Autodesk Inventor part; units mm, degrees
ref_plane "YZ Plane" through (0, 0, 0) normal (1, 0, 0) x (0, 1, 0)
ref_plane "XZ Plane" through (0, 0, 0) normal (0, 1, 0) x (-1, 0, 0)
ref_plane "XY Plane" through (0, 0, 0) normal (0, 0, 1) x (1, 0, 0)
sketch "Esquisse1" plane through (0, 0, 0) normal (0, 1, 0) x (-1, 0, 0)
  line L0 (28.5, 18.5) -> (-28.5, 18.5)
  line L1 (-28.5, 18.5) -> (-28.5, -18.5)
  line L2 (-28.5, -18.5) -> (28.5, -18.5)
  line L3 (28.5, -18.5) -> (28.5, 18.5)
  line L4 (28.5, 18.5) -> (-28.5, -18.5) construction
  line L5 (-28.5, 18.5) -> (28.5, -18.5) construction
  point P0 (0, 0)
  dimension "d0" = 57
  dimension "d1" = 37
extrude "Extrusion1" add sketch "Esquisse1" along normal blind 23
sketch "Esquisse2" plane through (0, 23, 0) normal (0, 1, 0) x (1, 0, 0)
  line L0 (-28.5, -18.5) -> (28.5, -18.5)
  line L1 (28.5, -18.5) -> (28.5, 18.5)
  line L2 (-28.5, 18.5) -> (-8.5, 18.5)
  line L3 (-8.5, 18.5) -> (-8.5, -18.5)
  line L4 (-8.5, -18.5) -> (-28.5, -18.5)
  line L5 (-28.5, -18.5) -> (-28.5, 18.5)
  line L6 (28.5, 18.5) -> (28.5, 16.5) construction
  line L7 (28.5, -18.5) -> (28.5, -16.5) construction
  line L8 (28.5, 16.5) -> (-8.5, 16.5)
  line L9 (-8.5, 16.5) -> (-8.5, -16.5)
  line L10 (-8.5, -16.5) -> (28.5, -16.5)
  line L11 (28.5, -16.5) -> (28.5, 16.5)
  point P0 (0, 0)
  dimension "d4" = 20
  dimension "d5" = 2
  dimension "d6" = 2
  dimension "d7" = 33
extrude "Extrusion2" cut sketch "Esquisse2" against normal blind 21 contours L3 L8 L1 L10
sketch "Esquisse3" plane through (-8.5, 23, 16.5) normal (1, 0, 0) x (0, 0, -1)
  line L0 (0, 0) -> (0, -21)
  line L1 (33, -21) -> (0, -21)
  line L2 (0, -21) -> (0, -2)
  line L3 (0, -2) -> (33, -2)
  line L4 (33, -2) -> (33, -21)
  point P0 (16.5, -23)
  dimension "d10" = 19
extrude "Extrusion3" cut sketch "Esquisse3" against normal blind 18
sketch "Esquisse4" plane through (-28.5, 0, -18.5) normal (-1, 0, 0) x (0, 0, 1)
  line L0 (37, 0) -> (18.5, 0) construction
  line L1 (18.5, 0) -> (18.5, 11.5) construction
  line L2 (18.5, 11.5) -> (37, 11.5) construction
  line L3 (37, 11.5) -> (37, 0) construction
  line L4 (6.5, 4.25) -> (30.5, 4.25)
  line L5 (30.5, 4.25) -> (30.5, 18.75)
  line L6 (30.5, 18.75) -> (6.5, 18.75)
  line L7 (6.5, 18.75) -> (6.5, 4.25)
  line L8 (6.5, 4.25) -> (30.5, 18.75) construction
  line L9 (30.5, 4.25) -> (6.5, 18.75) construction
  dimension "d13" = 18.5
  dimension "d14" = 11.5
  dimension "d15" = 24
  dimension "d16" = 14.5
extrude "Extrusion4" cut sketch "Esquisse4" against normal blind 5
properties part number "mount pour oeil"
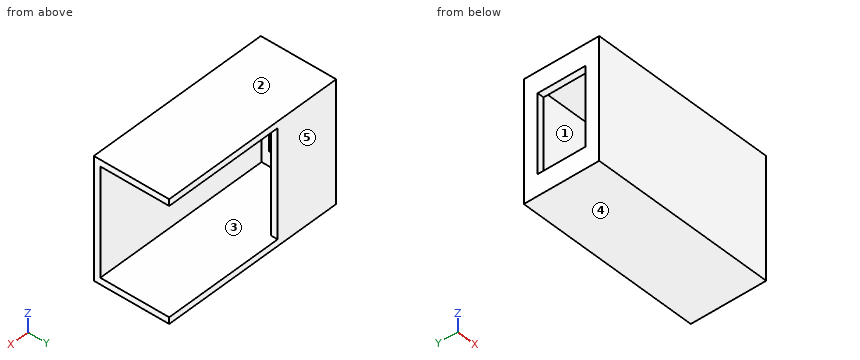
For this review, take the finished solid that the model builds, in its own axes (mm). Face numbers are marked on the shaded views. A direction names the side the tool comes from. Coordinates: 2 decimals unless noted, no trailing zeros. Loops run counter-clockwise (first coordinate to the right, second up) from the corner with the lowest first, then second, coordinate; pieces in that order, holes last. Notation, with made-up numbers: (-13, 83) -> (38, 83) arc R23 ccw to (38, 95) -> close; hole circle Ø11 at (-1, 12). An arc over 180 degrees is marked (long way). Return JSON: item names as keys, results as strings. Group by question number.
(1) Consider section A-A, the plane y = 14.75. Give the boundary of the cut face in (x, z).
(2) Tool access review of the marked faces 1 and 2: name each direction out of +Z, -Z, +X, -X, +Y, -Y from which nothing blocks a thin tool from reaching the whole face with its end or side.
(3) Consider section D-D, the plane z = 0. Give the boundary of the cut face in (x, y), plus the area to 3 significant figures.
(4) Consider section B-B, the plane z = -15. Give the boundary of the cut face in (x, y), plus the area to 3 significant figures.
(5) For pin 1 Ø2 at (x, z) = (0, 14.5) entering from +Y; pin 2 Ø0.6 at (y, z) = (21.5, 7) entering from +X, all flat-tipped, find the tip position at first contact; note any pin that passes through.
(6) To check wall thickness, follow L1, parallel to Z at x = 0.5, y = 19.5; L2, parallel to Y at x = -11.5, z = 9.5; L3, parallel to X at y = 20.5, z = -10. State the ranges of each line that lie inside material, in increasing order.
(7) Mouldability with a two-part tool opening along Z and no side actions: class the marked faces 3, 4 and 5 as pulls with the +Z half, pulls with the -Z half, needs draft (parallel to the pull), parting line crosses it, or undercut.
(8) Consider section C-C, the plane x = -13. Give the boundary of the cut face in (y, z), plus the area to 3 significant figures.
Results below:
{
 "1": {"outline": "(-28.5, -18.5) -> (28.5, -18.5) -> (28.5, -16.5) -> (-26.5, -16.5) -> (-26.5, -12) -> (-28.5, -12) -> close; (-28.5, 12) -> (-26.5, 12) -> (-26.5, 16.5) -> (28.5, 16.5) -> (28.5, 18.5) -> (-28.5, 18.5) -> close"},
 "2": {"face 1": "+X", "face 2": "+Z, +X, -X, +Y, -Y"},
 "3": {"outline": "(-28.5, 0) -> (28.5, 0) -> (28.5, 2) -> (-26.5, 2) -> (-26.5, 4.25) -> (-28.5, 4.25) -> close; (-28.5, 18.75) -> (-26.5, 18.75) -> (-26.5, 21) -> (-8.5, 21) -> (-8.5, 23) -> (-28.5, 23) -> close", "area": "163 mm2"},
 "4": {"outline": "(-28.5, 0) -> (28.5, 0) -> (28.5, 2) -> (-26.5, 2) -> (-26.5, 21) -> (-8.5, 21) -> (-8.5, 23) -> (-28.5, 23) -> close", "area": "192 mm2"},
 "5": {"pin 1": "stops at y = 2", "pin 2": "stops at x = -8.5"},
 "6": {"L1": "z = -18.5 to -16.5, 16.5 to 18.5", "L2": "y = 0 to 2, 21 to 23", "L3": "x = -28.5 to -26.5"},
 "7": {"face 3": "undercut", "face 4": "pulls with the -Z half", "face 5": "needs draft"},
 "8": {"outline": "(0, -18.5) -> (23, -18.5) -> (23, 18.5) -> (0, 18.5) -> close; hole (2, -16.5) -> (21, -16.5) -> (21, 16.5) -> (2, 16.5) -> close", "area": "224 mm2"}
}
